For this review, take the finished solid that the model builds, in its own axes (mm). Face numbers are marked on the shaded views. A direction names the side the tool comes from. Round coordinates to 2 decimals unless told otherwise and drop trailing zeros. Loops run counter-clockwise (first coordinate to the right, second up) from the corner with the lowest first, then second, coordinate; pieces in that order, holes last. Notation, with made-up numbers: M 83,12 L 102,12 A24 cw 102,40 Z; hole C 73,-1.75 d7. An arc over 180 degrees is marked long. One line per question, with ' | ' between items. Start each with the question number.
1) We need section C-C (z = 5.35). Give the boundary of the cut face in (x, y), and give its area (3 significant figures).
2) We need section B-B (y = 0.5). Give the boundary of the cut face in (x, z), and give its area (3 significant figures).
3) For the marked faces 5, 6 and 7, list the 3-axis set-ups (+Z, -Z, +X, -X, +Y, -Y) from which the entire face can be reached by the end or side of a thin tool; tool diameter is ignored.
4) We need section D-D (x = 1). Give the boundary of the cut face in (y, z).
5) We need section A-A (y = 4.25). Give the boundary of the cut face in (x, z), and give its area (3 significant figures).
6) For probe 1 along Z at (x, y) = (2.15, 3.85); probe 2 along Z at (x, y) = (-1, 0.5); probe 3 along X at (y, z) = (0.5, 0.5), list the stretches that pass through material, from the lowest coordinate up. Write a range as from..to.
7) Mouldability with a two-part tool opening along Z and no side actions: class the marked faces 1, 2, 3 and 4 as pulls with the +Z half, pulls with the -Z half, needs draft (parallel to the pull), parting line crosses it, or undercut.
8) For pin 1 Ø2 at (x, z) = (2.5, -1.5) entering from +Y; pin 2 Ø3 at (x, z) = (-3, 5.5) entering from -Y; pin 3 Ø0.8 at (x, z) = (2.5, 1) entering from +Y, all flat-tipped, find the tip position at first contact; note any pin that passes through.
```python
from build123d import *

# Parameters (mm, degrees)
SKETCH1_W               = 8
SKETCH1_H               = 5.2
SKETCH1_W_2             = 6.8
SKETCH1_H_2             = 4
BOSS_EXTRUDE1_DEPTH     = 2.5
SKETCH3_W               = 3.7
SKETCH3_H               = 9.55
SKETCH3_W_2             = 2.5
SKETCH3_H_2             = 8.35
BOSS_EXTRUDE2_DEPTH     = 3
SKETCH4_W               = 3.7
SKETCH4_H               = 4.95
BOSS_EXTRUDE3_DEPTH     = 0.6
SKETCH5_W               = 3.7
SKETCH5_H               = 9.55
BOSS_EXTRUDE4_DEPTH     = 0.6
SKETCH6_W               = 4.9
SKETCH6_H               = 5.2
BOSS_EXTRUDE5_DEPTH     = 0.6
FILLET2_R               = 0.7
SKETCH7_R               = 1
CUT_EXTRUDE1_DEPTH      = 4.5
CUT_EXTRUDE1_DRAFT      = -20
CUT_EXTRUDE3_REACH      = 10.671
SKETCH7_2_R             = 1
BOSS_EXTRUDE6_START     = -0.3
SKETCH8_R               = 1
BOSS_EXTRUDE6_DEPTH     = 1.6
BOSS_EXTRUDE6_DRAFT     = -1
CUT_EXTRUDE2_DEPTH      = 10.146720724
CUT_EXTRUDE2_DEPTH_BACK = 10.146720724
SKETCH9_R               = 0.75
FILLET3_R               = 0.5
FILLET5_R               = 0.5
FILLET6_R               = 0.5
CHAMFER1_SIZE           = 0.5
CHAMFER2_SIZE           = 0.2
CHAMFER2_SIZE2          = 0.357264117


# Read off the part's stored shape, not the designer's step: Boss-Extrude7
with BuildPart() as part:
    # Sketch1 → Boss-Extrude1 (new body)
    with BuildSketch(Plane(origin=(0, 0, 0), x_dir=(1, 0, 0), z_dir=(0, 1, 0))):
        Rectangle(SKETCH1_W, SKETCH1_H)
        Rectangle(SKETCH1_W_2, SKETCH1_H_2, mode=Mode.SUBTRACT)
    extrude(amount=BOSS_EXTRUDE1_DEPTH)

    # Sketch3 → Boss-Extrude2 (add)
    with BuildSketch(Plane(origin=(0, 2.5, 0), x_dir=(1, 0, 0), z_dir=(0, 1, 0))):
        with Locations((-2.15, -2.175)):
            Rectangle(SKETCH3_W, SKETCH3_H)
        with Locations((-2.15, -2.175)):
            Rectangle(SKETCH3_W_2, SKETCH3_H_2, mode=Mode.SUBTRACT)
    extrude(amount=BOSS_EXTRUDE2_DEPTH)

    # Sketch4 → Boss-Extrude3 (add)
    with BuildSketch(Plane.XZ.offset(-2.5)):
        with Locations((-2.15, 4.475)):
            Rectangle(SKETCH4_W, SKETCH4_H)
    extrude(amount=-BOSS_EXTRUDE3_DEPTH)

    # Sketch5 → Boss-Extrude4 (add)
    with BuildSketch(Plane(origin=(0, 5.5, 0), x_dir=(1, 0, 0), z_dir=(0, 1, 0))):
        with Locations((-2.15, -2.175)):
            Rectangle(SKETCH5_W, SKETCH5_H)
    extrude(amount=BOSS_EXTRUDE4_DEPTH)

    # Sketch6 → Boss-Extrude5 (add)
    with BuildSketch(Plane(origin=(0, 2.5, 0), x_dir=(1, 0, 0), z_dir=(0, 1, 0))):
        with Locations((1.55, 0)):
            Rectangle(SKETCH6_W, SKETCH6_H)
    extrude(amount=-BOSS_EXTRUDE5_DEPTH)

    # Fillet2
    fillet2_edges = [part.edges().sort_by_distance(p)[0] for p in [
        (-2.15, 5.5, -2),
        (-0.9, 5.5, 2.175),
        (-2.15, 5.5, 6.35),
        (-3.4, 5.5, 2.175),
    ]]
    fillet(fillet2_edges, radius=FILLET2_R)


with BuildPart() as cut_extrude1_tool:
    # Sketch7 → Cut-Extrude1 (with draft: the straight prism first)
    with BuildSketch(Plane.XZ.offset(-2.8)):
        with Locations((-2.15, 5.35)):
            Circle(SKETCH7_R)
    extrude(amount=CUT_EXTRUDE1_DEPTH)
    # Cut-Extrude1: the draft: its side faces are tilted about the plane it starts from
    cut_extrude1_sides = [cut_extrude1_tool.faces().sort_by_distance(p)[0] for p in [
        (-3.15, 0.55, 5.35),
    ]]
    draft(cut_extrude1_sides, Plane.XZ.offset(-2.8), CUT_EXTRUDE1_DRAFT)


with BuildPart() as part_1:
    add(part.part)

    # Cut-Extrude1: cut by cut_extrude1_tool
    add(cut_extrude1_tool.part, mode=Mode.SUBTRACT)

    # Sketch7<2> → Cut-Extrude3 (cut, up to next)
    with BuildSketch(Plane.XZ.offset(-2.8), mode=Mode.PRIVATE) as cut_extrude3_sk1:
        with Locations(Location((-2.15, 5.35, 0), (0, 0, 270))):
            Circle(SKETCH7_2_R)
    cut_extrude3_tool1 = extrude(cut_extrude3_sk1.sketch, amount=-CUT_EXTRUDE3_REACH, mode=Mode.PRIVATE) & part_1.part
    add(cut_extrude3_tool1.solids().sort_by_distance((-2.15, 2.8, 5.35))[0], mode=Mode.SUBTRACT)



with BuildPart() as body_2:
    # Sketch8 → Boss-Extrude6 (with draft: the straight prism first)
    with BuildSketch(Plane(origin=(0, 2.5, 0), x_dir=(-1, 0, 0), z_dir=(0, -1, 0)).offset(BOSS_EXTRUDE6_START)):
        with Locations((-2.15, -0.65)):
            Circle(SKETCH8_R)
    extrude(amount=-BOSS_EXTRUDE6_DEPTH)
    # Boss-Extrude6: the draft: its side faces are tilted about the plane it starts from
    boss_extrude6_sides = [body_2.faces().sort_by_distance(p)[0] for p in [
        (3.15, 3.6, 0.65),
    ]]
    draft(boss_extrude6_sides, Plane(origin=(0, 2.5, 0), x_dir=(-1, 0, 0), z_dir=(0, -1, 0)).offset(BOSS_EXTRUDE6_START), BOSS_EXTRUDE6_DRAFT)


with BuildPart() as part_2:
    add(part_1.part)

    add(body_2.part)  # Boss-Extrude7 merges body 2
    # Boss-Extrude7 outline → Boss-Extrude7 (revolve)
    with BuildSketch(Plane(origin=(2.15, 0, 0.65), x_dir=(1, 0, 0), z_dir=(0, 0, 1))):
        Polygon((1.010476231, 2.5), (1, 2.8), (0, 2.8), (0, 2.5), align=None)
    revolve(axis=Axis((2.15, 0, 0.65), (0, 1, 0)))

    # Sketch9 → Cut-Extrude2 (cut, two sides: drawn at the far end of the back side and taken through both)
    with BuildSketch(Plane(origin=(0, 4.4, 0), x_dir=(1, 0, 0), z_dir=(0, 1, 0)).offset(-CUT_EXTRUDE2_DEPTH_BACK)):
        with Locations(Location((2.15, -0.65, 0), (0, 0, 270))):
            Circle(SKETCH9_R)
    extrude(amount=CUT_EXTRUDE2_DEPTH + CUT_EXTRUDE2_DEPTH_BACK, mode=Mode.SUBTRACT)

    # Fillet3
    fillet3_edges = [part_2.edges().sort_by_distance(p)[0] for p in [
        (-4, 6.1, 2.175),
        (-2.15, 6.1, 6.95),
        (-0.3, 6.1, 2.175),
        (-2.15, 6.1, -2.6),
    ]]
    fillet(fillet3_edges, radius=FILLET3_R)

    # Fillet5
    # the kernel refuses this fillet: 0.5 mm, written as the material it takes off along each edge
    with BuildSketch(Plane(origin=(-0.8, 5.6, -2.1), x_dir=(1, 0, 0), z_dir=(0, 0, -1))) as fillet5_piece_1_section:
        Polygon((0, 0), (FILLET5_R, 0), (FILLET5_R, -FILLET5_R), (0, -FILLET5_R), align=None)
    fillet5_piece_1 = extrude(amount=FILLET5_R, mode=Mode.PRIVATE)
    fillet5_piece_1 = fillet5_piece_1 - Plane(origin=(-0.8, 5.6, -2.1), x_dir=(-0.7071067811865475, -0.7071067811865475, 0), z_dir=(0, 0, -1)) * Sphere(FILLET5_R, mode=Mode.PRIVATE)
    add(fillet5_piece_1, mode=Mode.SUBTRACT)
    with BuildSketch(Plane(origin=(-0.8, 5.6, 6.45), x_dir=(0, 0, 1), z_dir=(1, 0, 0))) as fillet5_piece_2_section:
        Polygon((0, 0), (FILLET5_R, 0), (FILLET5_R, -FILLET5_R), (0, -FILLET5_R), align=None)
    fillet5_piece_2 = extrude(amount=FILLET5_R, mode=Mode.PRIVATE)
    fillet5_piece_2 = fillet5_piece_2 - Plane(origin=(-0.8, 5.6, 6.45), x_dir=(0, -0.7071067811865475, -0.7071067811865475), z_dir=(1, 0, 0)) * Sphere(FILLET5_R, mode=Mode.PRIVATE)
    add(fillet5_piece_2, mode=Mode.SUBTRACT)
    with BuildSketch(Plane(origin=(-3.5, 5.6, -2.1), x_dir=(-1, 0, 0), z_dir=(0, 0, -1))) as fillet5_piece_3_section:
        Polygon((0, 0), (FILLET5_R, 0), (FILLET5_R, FILLET5_R), (0, FILLET5_R), align=None)
    fillet5_piece_3 = extrude(amount=FILLET5_R, mode=Mode.PRIVATE)
    fillet5_piece_3 = fillet5_piece_3 - Plane(origin=(-3.5, 5.6, -2.1), x_dir=(0.7071067811865475, -0.7071067811865475, 0), z_dir=(0, 0, -1)) * Sphere(FILLET5_R, mode=Mode.PRIVATE)
    add(fillet5_piece_3, mode=Mode.SUBTRACT)
    with BuildSketch(Plane(origin=(-3.5, 5.6, 6.45), x_dir=(0, 0, 1), z_dir=(-1, 0, 0))) as fillet5_piece_4_section:
        Polygon((0, 0), (FILLET5_R, 0), (FILLET5_R, FILLET5_R), (0, FILLET5_R), align=None)
    fillet5_piece_4 = extrude(amount=FILLET5_R, mode=Mode.PRIVATE)
    fillet5_piece_4 = fillet5_piece_4 - Plane(origin=(-3.5, 5.6, 6.45), x_dir=(0, -0.7071067811865475, -0.7071067811865475), z_dir=(-1, 0, 0)) * Sphere(FILLET5_R, mode=Mode.PRIVATE)
    add(fillet5_piece_4, mode=Mode.SUBTRACT)
    with BuildSketch(Plane(origin=(4, 3.75, 2.6), x_dir=(0, 0, -1), z_dir=(0, -1, 0)), Plane(origin=(4, 3.75, -2.6), x_dir=(-1, 0, 0), z_dir=(0, -1, 0))) as fillet5_piece_5:
        with BuildLine():
            CenterArc((FILLET5_R, -FILLET5_R), FILLET5_R, 90, 90)
            Line((0, -FILLET5_R), (0, 0))
            Line((0, 0), (FILLET5_R, 0))
        make_face()
    extrude(amount=5, mode=Mode.SUBTRACT)
    with BuildSketch(Plane(origin=(-4, 1.25, 6.95), x_dir=(0, 0, -1), z_dir=(0, 1, 0)), Plane(origin=(-0.3, 5.6, 6.95), x_dir=(0, 0, -1), z_dir=(0, -1, 0))) as fillet5_piece_6:
        with BuildLine():
            CenterArc((FILLET5_R, -FILLET5_R), FILLET5_R, 90, 90)
            Line((0, -FILLET5_R), (0, 0))
            Line((0, 0), (FILLET5_R, 0))
        make_face()
    extrude(amount=4.35, mode=Mode.SUBTRACT)
    with BuildSketch(Plane(origin=(-4, -1.25, -2.6), x_dir=(1, 0, 0), z_dir=(0, 1, 0))) as fillet5_piece_7:
        with BuildLine():
            CenterArc((FILLET5_R, -FILLET5_R), FILLET5_R, 90, 90)
            Line((0, -FILLET5_R), (0, 0))
            Line((0, 0), (FILLET5_R, 0))
        make_face()
    extrude(amount=6.85, mode=Mode.SUBTRACT)
    with BuildSketch(Plane(origin=(-0.3, 5.6, -2.6), x_dir=(-1, 0, 0), z_dir=(0, -1, 0))) as fillet5_piece_8:
        with BuildLine():
            CenterArc((FILLET5_R, -FILLET5_R), FILLET5_R, 90, 90)
            Line((0, -FILLET5_R), (0, 0))
            Line((0, 0), (FILLET5_R, 0))
        make_face()
    extrude(amount=3.1, mode=Mode.SUBTRACT)
    with BuildSketch(Plane(origin=(-4, -1.25, 2.6), x_dir=(0, 0, -1), z_dir=(0, 1, 0))) as fillet5_piece_9:
        with BuildLine():
            CenterArc((FILLET5_R, -FILLET5_R), FILLET5_R, 90, 90)
            Line((0, -FILLET5_R), (0, 0))
            Line((0, 0), (FILLET5_R, 0))
        make_face()
    extrude(amount=3.75, mode=Mode.SUBTRACT)

    # Fillet6
    # the kernel refuses this fillet: 0.5 mm, written as the material it adds along each edge
    with BuildSketch(Plane(origin=(-0.3, 2.5, 2.6), x_dir=(0, 1, 0), z_dir=(0, 0, -1))) as fillet6_piece_1:
        with BuildLine():
            CenterArc((FILLET6_R, FILLET6_R), FILLET6_R, 180, 90)
            Line((0, FILLET6_R), (0, 0))
            Line((0, 0), (FILLET6_R, 0))
        make_face()
    extrude(amount=4.7)
    with BuildSketch(Plane(origin=(-0.8, 2.5, -2.1), x_dir=(-0.5976672776328278, 0, 0.8017442392976482), z_dir=(0.8017442392976482, 0, 0.5976672776328278))) as fillet6_piece_2_section:
        with BuildLine():
            CenterArc((0.5 + FILLET6_R, -FILLET6_R), FILLET6_R, 90, 90)
            Line((0.5, -FILLET6_R), (0.5, 0))
            Line((0.5, 0), (0.5 + FILLET6_R, 0))
        make_face()
    fillet6_piece_2 = revolve(axis=Axis((-0.8, 2.5, -2.1), (0, -1, 0)), revolution_arc=233.296989237, mode=Mode.PRIVATE)
    fillet6_piece_2 = split(fillet6_piece_2, bisect_by=Plane(origin=(-0.425030478, 2.655814189, -2.6), z_dir=(0, 0, 1)), keep=Keep.TOP, mode=Mode.PRIVATE)
    fillet6_piece_2 = split(fillet6_piece_2, bisect_by=Plane(origin=(-0.425030478, 2.655814189, -2), z_dir=(0, 0, -1)), keep=Keep.TOP, mode=Mode.PRIVATE)
    add(fillet6_piece_2)

    # Chamfer1
    chamfer1_edges = [part_2.edges().sort_by_distance(p)[0] for p in [
        (-2.15, 3.1, 2),
    ]]
    chamfer(chamfer1_edges, length=CHAMFER1_SIZE)

    # Chamfer2
    chamfer2_edges = [part_2.edges().sort_by_distance(p)[0] for p in [
        (3.122071896, 4.4, 0.65),
    ]]
    chamfer2_side = [part_2.faces().sort_by_distance(p)[0] for p in [
        (3.094577551, 4.4, 0.65),
    ]]
    chamfer(chamfer2_edges, length=CHAMFER2_SIZE, length2=CHAMFER2_SIZE2, reference=chamfer2_side[0])


solid = part_2.part
```
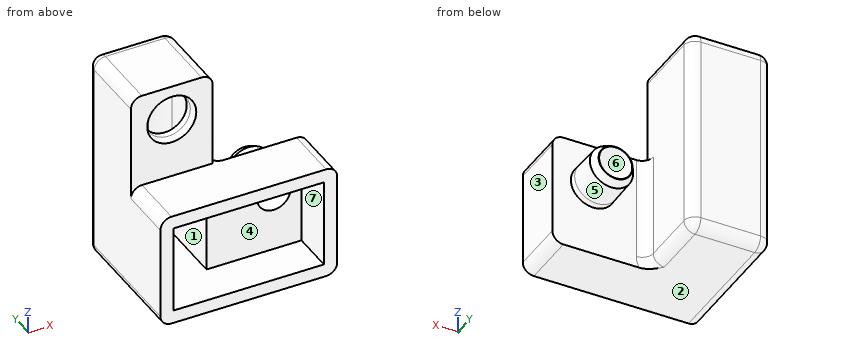
Answers below:
1) outline: M -4,2.5 L -3.26,2.5 L -3.15,2.8 L -3.15,3.1 L -3.4,3.1 L -3.4,4.8 A0.7 cw -2.7,5.5 L -1.6,5.5 A0.7 cw -0.9,4.8 L -0.9,3.1 L -1.15,3.1 L -1.15,2.8 L -1.04,2.5 L -0.3,2.5 L -0.3,5.6 A0.5 ccw -0.8,6.1 L -3.5,6.1 A0.5 ccw -4,5.6 Z | area: 6.19 mm^2
2) outline: M -4,-2.1 A0.5 ccw -3.5,-2.6 L 3.5,-2.6 A0.5 ccw 4,-2.1 L 4,2.1 A0.5 ccw 3.5,2.6 L -3.5,2.6 A0.5 ccw -4,2.1 Z; hole M -3.4,-2 L 3.4,-2 L 3.4,2 L -3.4,2 Z | area: 14.2 mm^2
3) face 5: +Y | face 6: +Y, -Y | face 7: -Y
4) outline: M 0,-2.6 L 2.5,-2.6 L 2.5,2.6 L 0,2.6 L 0,2 L 1.9,2 L 1.9,-2 L 0,-2 Z
5) outline: M -4,-2.1 A0.5 ccw -3.5,-2.6 L -0.8,-2.6 A0.5 ccw -0.3,-2.1 L -0.3,6.45 A0.5 ccw -0.8,6.95 L -3.5,6.95 A0.5 ccw -4,6.45 Z; C 2.15,0.65 d1.72; hole M -3.4,-2 L -0.9,-2 L -0.9,6.35 L -3.4,6.35 Z; hole C 2.15,0.65 d1.5 | area: 14.8 mm^2
6) probe 1: -0.33..-0.1, 1.4..1.63 | probe 2: -2.6..-2, 2..2.6 | probe 3: -4..-3.4, 3.4..4
7) face 1: undercut | face 2: pulls with the -Z half | face 3: needs draft | face 4: undercut
8) pin 1: y = 2.5 | pin 2: y = 2.5 | pin 3: y = 4.4
